```python
from build123d import *

# Parameters (mm, degrees)
F2_R = 0.99999


# Not quite as in the source:
# - a fillet or chamfer is up to 0.001 mm smaller than in the source, because OpenCascade refuses the exact size


with BuildPart() as f1:
    # F0 (on Front) → F1 (revolve)
    with BuildSketch(Plane.XZ):
        Polygon((0, 10), (0, 0), (20, 0), (20, 9.6603445709), (17, 9.6603445709), (17, 10.6603445709), (16, 10.6603445709), (16, 9.6603445709), (15, 9.6603445709), (15, 17.993060872), (13.75, 17.993060872), (13.75, 20), (11.25, 20), (11.25, 18), (10, 18), (10, 10), align=None)
    revolve(axis=Axis((10, 0, 0), (-1, 0, 0)))

    # F2 (radius 1 in the source; OpenCascade refuses exactly that, so slightly less here)
    f2_edges = [f1.edges().sort_by_distance(p)[0] for p in [
        (20, 0, -9.660345),
        (17, 0, -10.660345),
        (15, 0, -17.993061),
        (13.75, 0, -20),
    ]]
    fillet(f2_edges, radius=F2_R)


solid = f1.part
```
Work out the finished part from the listing and answer in its coordinate system (mm). A direction names the side the tool comes from. Coordinates: 2 decimals unless noted, no trailing zeros. Loops run counter-clockwise (first coordinate to the right, second up) from the corner with the lowest first, then second, coordinate; pieces in that order, holes last. Notation, with made-up numbers: (20.25, 4.25) - (34.25, 4.25) arc R19 cw to (34.25, 8.25) - close; hole circle Ø9 at (5.25, -14). An arc over 180 degrees is marked (long way). Use a Markdown table: item, result.
Item 1: Find section A-A, the plane x = 5.75. Determine the outline of the cut face in (y, z).
Evaluation:
| item | result |
|---|---|
| outline | circle Ø20 at (0, 0) |
Item 2: The mould has two halves that part along X. Classify faces 1 (the cylindrical face through (17.99, -8.57, 4.46)), 2 (the flat face through (16, 10, -2)), 3 (the flat face through (10, -8, 8)): +X half, -X half, draft (parallel to the pull), parting line (faces both ways), or undercut.
Evaluation:
| item | result |
|---|---|
| face 1 | draft |
| face 2 | undercut |
| face 3 | -X half |
Item 3: For faces 4 (the flat face through (20, 0, 0)), 5 (the cylindrical face through (15.49, -8.57, 4.46)), 6 (the flat face through (0, 0, 0)), 7 (the flat face through (13.75, -7, -17)), 8 (the flat face through (11.25, 3, -18)), determine the directions among +Z, -Z, +X, -X, +Y, -Y from which every point of the face is accessible in a straight line to the end or side of a thin tool.
Evaluation:
| item | result |
|---|---|
| face 4 | +Z, -Z, +X, +Y, -Y |
| face 5 | none |
| face 6 | +Z, -Z, -X, +Y, -Y |
| face 7 | +X |
| face 8 | -X |
Item 4: Consider probe 1 along X at (y, z) = (-2.5, -12); probe 2 along X at (y, z) = (2, 8.5); probe 3 along Y at (x, z) = (2.5, -3.5). Determine where each line is inside the solid, lowest interval first. Write a range as from..to.
Evaluation:
| item | result |
|---|---|
| probe 1 | x = 10..15 |
| probe 2 | x = 0..20 |
| probe 3 | y = -9.37..9.37 |
Item 5: Given pin 1 Ø4 at (x, y) = (7, 2.5) entering from +Z; pin 2 Ø2 at (x, z) = (8.5, 7) entering from -Y; pin 3 Ø1 at (y, z) = (-11.5, -10) entering from +X, each flat-ended and moving along its own axis, determine where each tip first touches the part or whether it passes through.
Evaluation:
| item | result |
|---|---|
| pin 1 | stops at z = 9.99 |
| pin 2 | stops at y = -8 |
| pin 3 | stops at x = 15 |
